from build123d import *

# Parameters (mm, degrees)
EXTRUDE_1_DEPTH     = 172
SHELL_START         = 6
SHELL_1_DEPTH       = 160
SKETCH_2_W          = 36
SKETCH_2_H          = 16
CUT_EXTRUDE_1_DEPTH = 74
EXTRUDE_2_DEPTH     = 2
SKETCH_4_R          = 10
CUT_EXTRUDE_2_DEPTH = 186
SKETCH_5_R          = 1.5
CUT_EXTRUDE_3_DEPTH = 10
EXTRUDE_3_DEPTH     = 172
SKETCH_7_W          = 36
SKETCH_7_H          = 16
CUT_EXTRUDE_4_DEPTH = 172
SKETCH_8_W          = 6
SKETCH_8_H          = 172
CUT_EXTRUDE_5_DEPTH = 3
EXTRUDE_4_DEPTH     = 15
CHAMFER_1_SIZE      = 15
CHAMFER_2_SIZE      = 15
CHAMFER_3_SIZE      = 8
SKETCH_10_R         = 1.35
CUT_EXTRUDE_6_DEPTH = 15
SKETCH_12_R         = 1.35
CUT_EXTRUDE_7_DEPTH = 15
CUT_EXTRUDE_8_DEPTH = 78
CUT_EXTRUDE_9_DEPTH = 78


# Read off the part's stored shape, not the designer's step: 抽壳1
with BuildPart() as part:
    # 草图1 → 凸台-拉伸1 (new body)
    with BuildSketch(Plane.XY):
        with BuildLine():
            Line((0, 0), (0, 40))
            Line((0, 40), (-5, 40))
            Line((-5, 40), (-5, 53))
            Line((-5, 53), (-23, 53))
            Line((-23, 53), (-64.888578151, 47.050698608))
            Line((-64.888578151, 47.050698608), (-15.121320344, -2.121320344))
            ThreePointArc((-15.121320344, -2.121320344), (-14.148050297, -2.771638598), (-13, -3))
            Line((-13, -3), (-5, -3))
            Line((-5, -3), (-5, 0))
            Line((-5, 0), (0, 0))
        make_face()
    extrude(amount=EXTRUDE_1_DEPTH)

    # 抽壳1 outline → 抽壳1 (cut)
    with BuildSketch(Plane.XY.offset(SHELL_START)):
        Polygon((-11, 6), (-6, 6), (-6, 34), (-11, 34), (-11, 47), (-22.576046832, 47), (-52.061983815, 42.812206246), (-11.767841448, 3), (-11, 3), align=None)
    extrude(amount=SHELL_1_DEPTH, mode=Mode.SUBTRACT)

    # 草图2 → 切除-拉伸1 (cut)
    with BuildSketch(Plane(origin=(0, 0, 0), x_dir=(0, 0, -1), z_dir=(1, 0, 0))):
        with Locations((-136, 10)):
            Rectangle(SKETCH_2_W, SKETCH_2_H)
        with Locations((-36, 10)):
            Rectangle(SKETCH_2_W, SKETCH_2_H)
    extrude(amount=-CUT_EXTRUDE_1_DEPTH, mode=Mode.SUBTRACT)

    # 草图3 → 凸台-拉伸2 (add, symmetric)
    with BuildSketch(Plane(origin=(0, 0, 86), x_dir=(-1, 0, 0), z_dir=(0, 0, -1))):
        Polygon((5, 53), (5, 40), (0, 40), (0, 0), (5, 0), (5, -3), (13, -3), (16.579355858, -0.680723591), (64.888578151, 47.050698608), (23, 53), align=None)
    extrude(amount=EXTRUDE_2_DEPTH, both=True)

    # 草图4 → 切除-拉伸2 (cut)
    with BuildSketch(Plane.XY.offset(172)):
        with Locations((-15, 21.071297481)):
            Circle(SKETCH_4_R)
    extrude(amount=-CUT_EXTRUDE_2_DEPTH, mode=Mode.SUBTRACT)

    # 草图5 → 切除-拉伸3 (cut)
    with BuildSketch(Plane(origin=(0, 53, 0), x_dir=(1, 0, 0), z_dir=(0, 1, 0))):
        with Locations(Location((-13.338195438, -63.5, 0), (0, 0, 270))):
            Circle(SKETCH_5_R)
        with Locations(Location((-13.338195438, -108.5, 0), (0, 0, 270))):
            Circle(SKETCH_5_R)
    extrude(amount=-CUT_EXTRUDE_3_DEPTH, mode=Mode.SUBTRACT)

    # 草图6 → 凸台-拉伸3 (add)
    with BuildSketch(Plane.XY.offset(172)):
        Polygon((-11, 6), (-14.804157153, 6), (-11.767841448, 3), (-11, 3), align=None)
    extrude(amount=-EXTRUDE_3_DEPTH)

    # 草图7 → 切除-拉伸4 (cut)
    with BuildSketch(Plane(origin=(0, 0, 0), x_dir=(0, 0, -1), z_dir=(1, 0, 0))):
        with Locations((-136, 10)):
            Rectangle(SKETCH_7_W, SKETCH_7_H)
        with Locations((-36, 10)):
            Rectangle(SKETCH_7_W, SKETCH_7_H)
    extrude(amount=-CUT_EXTRUDE_4_DEPTH, mode=Mode.SUBTRACT)

    # 草图8 → 切除-拉伸5 (cut)
    with BuildSketch(Plane.XZ.offset(3)):
        with Locations((-8, 86)):
            Rectangle(SKETCH_8_W, SKETCH_8_H)
    extrude(amount=-CUT_EXTRUDE_5_DEPTH, mode=Mode.SUBTRACT)

    # 草图9 → 凸台-拉伸4 (add)
    with BuildSketch(Plane(origin=(0, 0, 0), x_dir=(0, 0, -1), z_dir=(1, 0, 0))):
        Polygon((-86, 40), (-151, 40), (-151, 35), (-86, 35), (-21, 35), (-21, 40), align=None)
    extrude(amount=EXTRUDE_4_DEPTH)

    # 倒角1
    chamfer_1_edges = [part.edges().sort_by_distance(p)[0] for p in [
        (15, 37.5, 151),
    ]]
    chamfer(chamfer_1_edges, length=CHAMFER_1_SIZE - 0.0001)  # a hair under: the kernel refuses the full size

    # 倒角2
    chamfer_2_edges = [part.edges().sort_by_distance(p)[0] for p in [
        (15, 37.5, 21),
    ]]
    chamfer(chamfer_2_edges, length=CHAMFER_2_SIZE - 0.0001)  # a hair under: the kernel refuses the full size

    # 倒角3
    chamfer_3_edges = [part.edges().sort_by_distance(p)[0] for p in [
        (0, 35, 86),
    ]]
    chamfer(chamfer_3_edges, length=CHAMFER_3_SIZE)

    # 草图10 → 切除-拉伸6 (cut)
    with BuildSketch(Plane.XZ):
        with Locations((-5, 158)):
            Circle(SKETCH_10_R)
        with Locations((-5, 111)):
            Circle(SKETCH_10_R)
        with Locations((-5, 61)):
            Circle(SKETCH_10_R)
        with Locations((-5, 14.01360213)):
            Circle(SKETCH_10_R)
    extrude(amount=-CUT_EXTRUDE_6_DEPTH, mode=Mode.SUBTRACT)

    # 草图12 → 切除-拉伸7 (cut)
    with BuildSketch(Plane(origin=(0, 40, 0), x_dir=(1, 0, 0), z_dir=(0, 1, 0))):
        with Locations(Location((5, -41, 0), (0, 0, 270))):
            Circle(SKETCH_12_R)
        with Locations(Location((5, -86, 0), (0, 0, 270))):
            Circle(SKETCH_12_R)
        with Locations(Location((5, -131, 0), (0, 0, 270))):
            Circle(SKETCH_12_R)
    extrude(amount=-CUT_EXTRUDE_7_DEPTH, mode=Mode.SUBTRACT)

    # 草图14 → 切除-拉伸8 (cut)
    with BuildSketch(Plane(origin=(0, 0, 84), x_dir=(-1, 0, 0), z_dir=(0, 0, -1))):
        Polygon((11, 47), (6, 34), (11, 34), align=None)
    extrude(amount=CUT_EXTRUDE_8_DEPTH, mode=Mode.SUBTRACT)

    # 草图16 → 切除-拉伸9 (cut)
    with BuildSketch(Plane.XY.offset(88)):
        Polygon((-11, 47), (-11, 34), (-6, 34), align=None)
    extrude(amount=CUT_EXTRUDE_9_DEPTH, mode=Mode.SUBTRACT)


solid = part.part
Here's how the part is built. I have some questions about the finished solid (model axes, mm). A direction names the side the tool comes from. Coordinates: 2 decimals unless noted, no trailing zeros. Loops run counter-clockwise (first coordinate to the right, second up) from the corner with the lowest first, then second, coordinate; pieces in that order, holes last. Notation, with made-up numbers: (-28, -36.75) -> (18, -36.75) arc R22 ccw to (18, -1.75) -> close; hole circle Ø7 at (41.5, 33.25). An arc over 180 degrees is marked (long way). Use one line per item in the form item = value. Start each with the question number.
(1) If we section it at B-B (y = 45): Please give me the cut outline in (x, z).
(2) If we section it at C-C (z = 120): Please give me the cut outline in (x, y), then the cut area to 3 significant figures.
(3) Will these pins go through, and if not, where does the flat tip stop? pin 1 (6 mm diameter, centred on y = 32.5, z = 99, fed in from -X); pin 2 (7.5 mm diameter, centred on x = 11, z = 106, fed in from -Y); pin 3 (5.5 mm diameter, centred on y = 9, z = 163, fed in from -X).
(4) We'd pull the mould along Z, two halves only. Please class faces 1 (the face through (6, 36, 145)), 2 (the face through (-24, 36, 166)), 3 (the face through (-26, 32, 0)), 4 (the face through (-8.535, 40.591, 45.546)): pulls with the +Z half, pulls with the -Z half, needs draft (parallel to the pull), parting line crosses it, or undercut.
(5) If we section it at D-D (x = -56): Please give me the cut outline in (y, z).
(6) If we section it at A-A (z = 75): Please give me the cut outline in (x, y), then the cut area to 3 significant figures.
(7) On a 3-axis mill with a long thin cutter (end or side, diameter ignored), from which of +Z, -Z, +X, -X, +Y, -Y can I reach the whole of each face in a straight line? I mean faces 5 (the face through (-3, 18, 136)), 6 (the face through (-10, 6, 103)), 7 (the face through (-12.89, 50.04, 64.93)), 8 (the face through (-5, 0, 85)). Say none if no direction works.
(8) Please list where these lines run through material, in increasing order: line 1 along Z through (x, y) = (-27, 21); line 2 along X through (y, z) = (37.75, 41); line 3 along Z through (x, y) = (5, 34.5).
Verdict:
q1.outline = (-62.81, 0) -> (-5, 0) -> (-5, 172) -> (-62.81, 172) -> close; hole (-36.66, 6) -> (-10.23, 6) -> (-10.23, 84) -> (-36.66, 84) -> close; hole (-36.66, 88) -> (-10.23, 88) -> (-10.23, 166) -> (-36.66, 166) -> close
q2.outline = (-64.89, 47.05) -> (-35.49, 18) -> (-26.95, 18) -> (-52.06, 42.81) -> (-22.58, 47) -> (-11, 47) -> (-6, 34) -> (-6, 25.43) arc R10 cw to (-5.48, 18) -> (0, 18) -> (0, 27) -> (8, 35) -> (15, 35) -> (15, 40) -> (-5, 40) -> (-5, 53) -> (-23, 53) -> close; (-19.29, 2) -> (-15.12, -2.12) arc R3 ccw to (-13, -3) -> (-11, -3) -> (-11, 0) -> (0, 0) -> (0, 2) -> close
q2.area = 877 mm²
q3.pin_1 = -53.2
q3.pin_2 = 34.25
q3.pin_3 = -29.16
q4.face_1 = pulls with the +Z half
q4.face_2 = undercut
q4.face_3 = pulls with the -Z half
q4.face_4 = undercut
q5.outline = (38.27, 0) -> (48.31, 0) -> (48.31, 172) -> (38.27, 172) -> close
q6.outline = (-64.89, 47.05) -> (-15.12, -2.12) arc R3 ccw to (-13, -3) -> (-11, -3) -> (-11, 0) -> (0, 0) -> (0, 27) -> (8, 35) -> (15, 35) -> (15, 40) -> (-5, 40) -> (-5, 53) -> (-23, 53) -> close; hole (-52.06, 42.81) -> (-14.8, 6) -> (-6, 6) -> (-6, 16.71) arc R10 ccw to (-6, 25.43) -> (-6, 34) -> (-11, 47) -> (-22.58, 47) -> close
q6.area = 1,140 mm²
q7.face_5 = +X, -X
q7.face_6 = none
q7.face_7 = +Y
q7.face_8 = +Z, -Z, +X, -Y
q8.line_1 = 0 to 6, 84 to 88, 166 to 172
q8.line_2 = -55.48 to -46.94, -7.44 to 3.65, 6.35 to 15
q8.line_3 = 26 to 39.65, 42.35 to 84.65, 87.35 to 129.65, 132.35 to 146
